```python
from build123d import *

# Parameters (mm, degrees)
SKETCH5_W           = 150
SKETCH5_H           = 150
CUT_EXTRUDE1_DEPTH  = 100
SKETCH6_W           = 100
SKETCH6_H           = 100
BOSS_EXTRUDE1_DEPTH = 1000


with BuildPart() as part:
    # Sketch1 → Loft1 section 0
    with BuildSketch(Plane(origin=(0, 0, 0), x_dir=(1, 0, 0), z_dir=(0, 1, 0)), mode=Mode.PRIVATE) as loft1_s0:
        with BuildLine():
            Line((-500, -500), (500, -500))
            Line((500, -500), (500, 500))
            Line((500, 500), (-500, 500))
            Line((-500, 500), (-500, -500))
        make_face()
    loft([loft1_s0.sketch, Vertex(0, -400, 0)])

    # Sketch5 → Cut-Extrude1 (cut)
    with BuildSketch(Plane(origin=(0, -400, 0), x_dir=(-1, 0, 0), z_dir=(0, -1, 0))):
        Rectangle(SKETCH5_W, SKETCH5_H)
    extrude(amount=-CUT_EXTRUDE1_DEPTH, mode=Mode.SUBTRACT)

    # Sketch6 → Boss-Extrude1 (add)
    with BuildSketch(Plane(origin=(0, 0, 0), x_dir=(1, 0, 0), z_dir=(0, 1, 0))):
        with Locations((-450, 450)):
            Rectangle(SKETCH6_W, SKETCH6_H)
        with Locations((450, 450)):
            Rectangle(SKETCH6_W, SKETCH6_H)
        with Locations((-450, -450)):
            Rectangle(SKETCH6_W, SKETCH6_H)
        with Locations((450, -450)):
            Rectangle(SKETCH6_W, SKETCH6_H)
    extrude(amount=-BOSS_EXTRUDE1_DEPTH)


solid = part.part
```
Verification items for the finished model (mm, model axes). A direction names the side the tool comes from. Coordinates: 2 decimals unless noted, no trailing zeros. Order: outer loops, then holes, each group sorted by start corner. A loop starts at its lowest first (then second) coordinate and runs counter-clockwise, first axis right, second up. Notation, with made-up numbers: (76.5, 69) -> (106.5, 69) arc R37 ccw to (106.5, 107) -> close; hole circle Ø3 at (12.25, 36.25). An arc over 180 degrees is marked (long way). Answer as CSV lines item,"result". Start each with the question number.
1) Cross-section at D-D, the plane x = -284.5. Record the boundary of the cut face in (y, z), then the cut area to 3 significant figures.
2) Cross-section at B-B, the plane y = -821.5. Record the boundary of the cut face in (x, z), then the cut area to 3 significant figures.
3) Set-up check for faces 1 (the face through (331.75, -134.6, 5.6)), 2 (the face through (-75, -320, 1)), 3 (the face through (0, 0, 14)): record each of +Z, -Z, +X, -X, +Y, -Y from which the full face is reachable in a straight line by a thin tool's end or side.
4) Release check for a two-part mould opening along Z. For faces 4 (the face through (500, -493, -449)), 5 (the face through (1, -300, -1)), 6 (the face through (5.6, -134.6, -331.75)) record: released by +Z, released by -Z, zero draft, split by the parting line, or undercut.
5) Material ranges on L1, parallel to Z at x = -457.5, y = -239; L2, parallel to Y at x = 30, z = 44; L3, parallel to Y at x = 10, z = 175, recorded low to high. Write a range as [from, to].
6) Cross-section at C-C, the plane z = 193. Record the boundary of the cut face in (x, y).
7) Gauge pin test, flat ends, axial feed: pin 1 Ø10 at (x, z) = (-316, 62) entering from +Y; pin 2 Ø12 at (y, z) = (-315, 1.5) entering from -X; pin 3 Ø3 at (x, z) = (340, 5) entering from -Y. Record the tip position at first contact, or that the pin passes through.
8) Cross-section at A-A, the plane y = -203. Record the boundary of the cut face in (x, z), then the cut area to 3 significant figures.
Conclusion:
1,outline,"(-172.4, -284.5) -> (0, -500) -> (0, 500) -> (-172.4, 284.5) -> close"
1,area,"135,000 mm²"
2,outline,"(-500, -500) -> (-400, -500) -> (-400, -400) -> (-500, -400) -> close; (-500, 400) -> (-400, 400) -> (-400, 500) -> (-500, 500) -> close; (400, -500) -> (500, -500) -> (500, -400) -> (400, -400) -> close; (400, 400) -> (500, 400) -> (500, 500) -> (400, 500) -> close"
2,area,"40,000 mm²"
3,face 1,"+X, -Y"
3,face 2,"-Y"
3,face 3,"+Z, -Z, +X, -X, +Y"
4,face 4,"zero draft"
4,face 5,"undercut"
4,face 6,"released by -Z"
5,L1,"z = [-500, -400], [400, 500]"
5,L2,"y = [-300, 0]"
5,L3,"y = [-260, 0]"
6,outline,"(-500, 0) -> (-193, -245.6) -> (193, -245.6) -> (500, 0) -> close"
7,pin 1,"stops at y = 0"
7,pin 2,"stops at x = -113.75"
7,pin 3,"stops at y = -129.2"
8,outline,"(-500, -500) -> (-400, -500) -> (-400, -400) -> (-500, -400) -> close; (-500, 400) -> (-400, 400) -> (-400, 500) -> (-500, 500) -> close; (-246.25, -246.25) -> (246.25, -246.25) -> (246.25, 246.25) -> (-246.25, 246.25) -> close; (400, -500) -> (500, -500) -> (500, -400) -> (400, -400) -> close; (400, 400) -> (500, 400) -> (500, 500) -> (400, 500) -> close"
8,area,"283,000 mm²"
